```python
from build123d import *

# Parameters (mm, degrees)
SKETCH1_R           = 1.75
BOSS_EXTRUDE1_DEPTH = 2
SKETCH2_W           = 9.5
SKETCH2_H           = 4.5
BOSS_EXTRUDE2_DEPTH = 9.5


with BuildPart() as part:
    # Sketch1 → Boss-Extrude1 (new body)
    with BuildSketch(Plane(origin=(0, 0, 0), x_dir=(1, 0, 0), z_dir=(0, 1, 0))):
        Polygon((17.25, 4.5), (13.25, 4.5), (13.25, -4.5), (17.25, -4.5), (17.25, -7.5), (-17.25, -7.5), (-17.25, 7.5), (17.25, 7.5), align=None)
        with Locations((-8.25, 0)):
            Circle(SKETCH1_R, mode=Mode.SUBTRACT)
    extrude(amount=BOSS_EXTRUDE1_DEPTH)

    # Sketch2 → Boss-Extrude2 (add)
    with BuildSketch(Plane(origin=(0, 2, 0), x_dir=(1, 0, 0), z_dir=(0, 1, 0))):
        with Locations((1, 4.75)):
            Rectangle(SKETCH2_W, SKETCH2_H)
    extrude(amount=BOSS_EXTRUDE2_DEPTH)


solid = part.part
```
Check sheet for the modelled part. Datum: model origin and axes. Units: mm. A direction names the side the tool comes from. Coordinates: 2 decimals unless noted, no trailing zeros. Write each loop counter-clockwise with the first axis right and the second up, starting at its lowest first coordinate (ties: lowest second). Pieces come first, ordered by that corner, then holes. Notation, with made-up numbers: (87, 36) -> (143, 36) arc R13 ccw to (143, 50) -> close; hole circle Ø7 at (17.25, -38.75). An arc over 180 degrees is marked (long way). Use a Markdown table: item, result.
1. Sectioned sample at A-A (x = -8.25). Enter the section's corners in (y, z), plus the area to 3 significant figures.
Reported:
| item | result |
|---|---|
| outline | (0, -7.5) -> (2, -7.5) -> (2, -1.75) -> (0, -1.75) -> close; (0, 1.75) -> (2, 1.75) -> (2, 7.5) -> (0, 7.5) -> close |
| area | 23.0 mm2 |
2. Sectioned sample at D-D (z = -5.75). Enter the section's corners in (x, y), plus the area to 3 significant figures.
Reported:
| item | result |
|---|---|
| outline | (-17.25, 0) -> (17.25, 0) -> (17.25, 2) -> (5.75, 2) -> (5.75, 11.5) -> (-3.75, 11.5) -> (-3.75, 2) -> (-17.25, 2) -> close |
| area | 159 mm2 |
3. Tool access check on faces 1 (the flat face through (15, 1, 4.5)), 2 (the flat face through (1, 7, -7)), 3 (the flat face through (-3.75, 7, -5)), 4 (the flat face through (5.75, 7, -5)), 5 (the flat face through (1, 7, -2.5)). Record the directions out of +Z, -Z, +X, -X, +Y, -Y that give a thin tool (end or side, any length) a straight path to the whole face; none if there is none.
Reported:
| item | result |
|---|---|
| face 1 | +X, +Y, -Y |
| face 2 | -Z, +X, -X, +Y |
| face 3 | +Z, -Z, -X, +Y |
| face 4 | +Z, -Z, +X, +Y |
| face 5 | +Z, +X, -X, +Y |
4. Sectioned sample at C-C (y = 1). Enter the section's corners in (x, z), plus the area to 3 significant figures.
Reported:
| item | result |
|---|---|
| outline | (-17.25, -7.5) -> (17.25, -7.5) -> (17.25, -4.5) -> (13.25, -4.5) -> (13.25, 4.5) -> (17.25, 4.5) -> (17.25, 7.5) -> (-17.25, 7.5) -> close; hole circle Ø3.5 at (-8.25, 0) |
| area | 472 mm2 |
5. Sectioned sample at B-B (z = 0). Enter the section's corners in (x, y).
Reported:
| item | result |
|---|---|
| outline | (-17.25, 0) -> (-10, 0) -> (-10, 2) -> (-17.25, 2) -> close; (-6.5, 0) -> (13.25, 0) -> (13.25, 2) -> (-6.5, 2) -> close |
6. Go/stop test with flat-tipped pins: pin 1 Ø7.5 at (x, z) = (6, 3.5) entering from +Y; pin 2 Ø5 at (x, y) = (3, 7) entering from -Z; pin 3 Ø3 at (x, y) = (0.5, 6.5) entering from +Z. Record where each tip stops, or that it passes through.
Reported:
| item | result |
|---|---|
| pin 1 | stops at y = 2 |
| pin 2 | stops at z = -7 |
| pin 3 | stops at z = -2.5 |
7. Scan lines: line 1 along X through (y, z) = (0.95, 0); line 2 along Z through (x, y) = (-8.25, 1.1); line 3 along Z through (x, y) = (3, 2.25). Record each from-to range of solid material in increasing order.
Reported:
| item | result |
|---|---|
| line 1 | x = -17.25 to -10, -6.5 to 13.25 |
| line 2 | z = -7.5 to -1.75, 1.75 to 7.5 |
| line 3 | z = -7 to -2.5 |
